from build123d import *

# Parameters (mm, degrees)
BOSS_EXTRUDE1_DEPTH = 4.7625
BOSS_EXTRUDE2_DEPTH = 12.7
SKETCH6_R           = 2.1
BOSS_EXTRUDE3_DEPTH = 6.35
CUT_EXTRUDE1_DEPTH  = 3.175
CUT_EXTRUDE2_DEPTH  = 3.175
FILLET1_R           = 5.08


with BuildPart() as part:
    # Sketch1 → Boss-Extrude1 (new body)
    with BuildSketch(Plane(origin=(0, 0, 0), x_dir=(1, 0, 0), z_dir=(0, 1, 0))):
        with BuildLine():
            Line((-22.225, -19.05), (22.225, -19.05))
            ThreePointArc((22.225, -19.05), (26.715128061, -17.190128061), (28.575, -12.7))
            Line((28.575, -12.7), (28.575, 12.7))
            ThreePointArc((28.575, 12.7), (26.715128061, 17.190128061), (22.225, 19.05))
            Line((22.225, 19.05), (-22.225, 19.05))
            ThreePointArc((-22.225, 19.05), (-26.715128061, 17.190128061), (-28.575, 12.7))
            Line((-28.575, 12.7), (-28.575, -12.7))
            ThreePointArc((-28.575, -12.7), (-26.715128061, -17.190128061), (-22.225, -19.05))
        make_face()
    extrude(amount=BOSS_EXTRUDE1_DEPTH)

    # Sketch2 → Boss-Extrude2 (add)
    with BuildSketch(Plane(origin=(0, 4.7625, 0), x_dir=(1, 0, 0), z_dir=(0, 1, 0))):
        with BuildLine():
            Line((-22.225, -19.05), (22.225, -19.05))
            ThreePointArc((22.225, -19.05), (26.715128061, -17.190128061), (28.575, -12.7))
            Line((28.575, -12.7), (28.575, 12.7))
            ThreePointArc((28.575, 12.7), (26.715128061, 17.190128061), (22.225, 19.05))
            Line((22.225, 19.05), (-22.225, 19.05))
            ThreePointArc((-22.225, 19.05), (-26.715128061, 17.190128061), (-28.575, 12.7))
            Line((-28.575, 12.7), (-28.575, -12.7))
            ThreePointArc((-28.575, -12.7), (-26.715128061, -17.190128061), (-22.225, -19.05))
        make_face()
        with BuildLine():
            Line((-22.225, -15.875), (22.225, -15.875))
            ThreePointArc((22.225, -15.875), (24.47006403, -14.94506403), (25.4, -12.7))
            Line((25.4, -12.7), (25.4, 12.7))
            ThreePointArc((25.4, 12.7), (24.47006403, 14.94506403), (22.225, 15.875))
            Line((22.225, 15.875), (-22.225, 15.875))
            ThreePointArc((-22.225, 15.875), (-24.47006403, 14.94506403), (-25.4, 12.7))
            Line((-25.4, 12.7), (-25.4, -12.7))
            ThreePointArc((-25.4, -12.7), (-24.47006403, -14.94506403), (-22.225, -15.875))
        make_face(mode=Mode.SUBTRACT)
    extrude(amount=BOSS_EXTRUDE2_DEPTH)

    # Sketch6 → Boss-Extrude3 (add)
    with BuildSketch(Plane.XZ):
        with BuildLine():
            Line((4.370745694, -27.291557117), (7.9375, -19.05))
            Line((7.9375, -19.05), (-7.9375, -19.05))
            Line((-7.9375, -19.05), (-4.370745694, -27.291557117))
            ThreePointArc((-4.370745694, -27.291557117), (0, -30.1625), (4.370745694, -27.291557117))
        make_face()
        with Locations((0, -25.4)):
            Circle(SKETCH6_R, mode=Mode.SUBTRACT)
    boss_extrude3 = extrude(amount=-BOSS_EXTRUDE3_DEPTH)

    # Sketch4 → Cut-Extrude1 (cut)
    with BuildSketch(Plane.ZY.offset(28.575)):
        with BuildLine():
            Line((-5.2705, 3.8989), (5.2705, 3.8989))
            ThreePointArc((5.2705, 3.8989), (6.168525612, 4.270874388), (6.5405, 5.1689))
            Line((6.5405, 5.1689), (6.5405, 10.2489))
            ThreePointArc((6.5405, 10.2489), (6.168525612, 11.146925612), (5.2705, 11.5189))
            Line((5.2705, 11.5189), (-5.2705, 11.5189))
            ThreePointArc((-5.2705, 11.5189), (-6.168525612, 11.146925612), (-6.5405, 10.2489))
            Line((-6.5405, 10.2489), (-6.5405, 5.1689))
            ThreePointArc((-6.5405, 5.1689), (-6.168525612, 4.270874388), (-5.2705, 3.8989))
        make_face()
    extrude(amount=-CUT_EXTRUDE1_DEPTH, mode=Mode.SUBTRACT)

    # Sketch5 → Cut-Extrude2 (cut)
    with BuildSketch(Plane(origin=(28.575, 0, 0), x_dir=(0, 0, -1), z_dir=(1, 0, 0))):
        with BuildLine():
            Line((-7.112, 5.1689), (7.112, 5.1689))
            ThreePointArc((7.112, 5.1689), (8.010025612, 5.540874388), (8.382, 6.4389))
            Line((8.382, 6.4389), (8.382, 13.5509))
            ThreePointArc((8.382, 13.5509), (8.010025612, 14.448925612), (7.112, 14.8209))
            Line((7.112, 14.8209), (-7.112, 14.8209))
            ThreePointArc((-7.112, 14.8209), (-8.010025612, 14.448925612), (-8.382, 13.5509))
            Line((-8.382, 13.5509), (-8.382, 6.4389))
            ThreePointArc((-8.382, 6.4389), (-8.010025612, 5.540874388), (-7.112, 5.1689))
        make_face()
    extrude(amount=-CUT_EXTRUDE2_DEPTH, mode=Mode.SUBTRACT)

    # Mirror3: Boss-Extrude3 across plane
    add(boss_extrude3.mirror(Plane.XY))

    # Fillet1
    fillet1_edges = [part.edges().sort_by_distance(p)[0] for p in [
        (7.9375, 3.175, 19.05),
        (-7.9375, 3.175, 19.05),
        (-7.9375, 3.175, -19.05),
        (7.9375, 3.175, -19.05),
    ]]
    fillet(fillet1_edges, radius=FILLET1_R)


solid = part.part
Verification items for the finished model (mm, model axes). A direction names the side the tool comes from. Round coordinates to 2 decimals unless told otherwise and drop trailing zeros. Loops run counter-clockwise (first coordinate to the right, second up) from the corner with the lowest first, then second, coordinate; pieces in that order, holes last. Notation, with made-up numbers: M 35,88.5 L 71,88.5 A12 ccw 71,96.5 Z; hole C 71,-13 d1. An arc over 180 degrees is marked long. Write each question's results on one line, items separated by ' | '.
1) Section check B-B on x = 0. State how many separate pieces and enclosed holes the cut face has, then the cut area to 3 significant figures.
Checks:
separate pieces: 3 | enclosed holes: 0 | area: 350 mm2
2) Mould release check, pull along Z, two halves, no side actions. Record for faces 6 (the flat face through (-27, 11.519, 0)), 7 (the flat face through (0, 0, 0)), 8 (the cylindrical face through (-26.764, 8.609, 17.14)): released by +Z, released by -Z, zero draft, split by the parting line, or undercut.
Checks:
face 6: undercut | face 7: zero draft | face 8: released by +Z
3) Access from +Z, -Z, +X, -X, +Y, -Y to the whole of each face (thin tool, end or side, straight path). Record for faces 1 (the flat face through (27, 14.821, 0)), 2 (the flat face through (-27, 8, -6.54)), 3 (the cylindrical face through (-24.445, 11.024, -14.97)), 4 (the cylindrical face through (-8.52, 3.22, -19.86)), 5 (the cylindrical face through (-8.52, 3.22, 19.86)).
Checks:
face 1: +X | face 2: +X, -X | face 3: +Y | face 4: -Z, -X, +Y, -Y | face 5: +Z, -X, +Y, -Y
4) Scan lines: L1, parallel to X at y = 13.75, z = -9 (3 decimals); L2, parallel to Z at x = 0, y = 2.25; L3, parallel to Z at x = 15.5, y = 15.75 (3 decimals). Record each from-to range of solid material in increasing order. Write a range as from..to.
Checks:
L1: x = -28.575..-25.4, 25.4..28.575 | L2: z = -30.16..-27.5, -23.3..23.3, 27.5..30.16 | L3: z = -19.05..-15.875, 15.875..19.05
5) Gauge pin test, flat ends, axial feed: P1, Ø2.5, axis at x = -26.5, y = 8, coming from the +Z side; P2, Ø6.5, axis at x = -5.5, y = 13.5, coming from the -Z side; P3, Ø9, axis at x = 3, z = 27, coming from the +Y side. Record the tip position at first contact, or that the pin passes through.
Checks:
P1: stops at z = 18.28 | P2: stops at z = -19.05 | P3: stops at y = 6.35
6) Section check C-C on z = -25.4. Record the boundary of the cut face in (x, y).
Checks:
outline: M -5.19,0 L -2.1,0 L -2.1,6.35 L -5.19,6.35 Z; M 2.1,0 L 5.19,0 L 5.19,6.35 L 2.1,6.35 Z
